The listing builds one solid part. Answer for the finished solid, in the listing's coordinates (mm). A direction names the side the tool comes from. Round coordinates to 2 decimals unless told otherwise and drop trailing zeros. Order: outer loops, then holes, each group sorted by start corner. A loop starts at its lowest first (then second) coordinate and runs counter-clockwise, first axis right, second up. Notation, with made-up numbers: (-23, 9) - (-16, 9) arc R19 cw to (-16, 13) - close; hole circle Ø9 at (-4.5, 13). An arc over 180 degrees is marked (long way). Write item = value, one per line.
from build123d import *

# Parameters (mm, degrees)
F0_R      = 2.25
F1_DEPTH  = 10
F3_DEPTH  = 20
F4_R      = 2.25
F5_DEPTH  = 5
F6_R      = 2.01
F7_DEPTH  = 5
F8_R      = 3.75
F9_DEPTH  = 2
F10_R     = 3.75
F11_DEPTH = 2


with BuildPart() as f1:
    # F0 (on Top) → F1 (new body)
    with BuildSketch(Plane.XY):
        Polygon((28.65822, 18.559446), (28.65822, -1.440554), (48.65822, -1.440554), (68.65822, -21.440554), (88.65822, -21.440554), (88.65822, -1.440554), (68.65822, -1.440554), (68.65822, 18.559446), align=None)
        with Locations((43.65822, 8.559446)):
            Circle(F0_R, mode=Mode.SUBTRACT)
        with Locations((58.65822, 8.559446)):
            Circle(F0_R, mode=Mode.SUBTRACT)
    extrude(amount=F1_DEPTH)

    # F2 (on face) → F3 (join)
    with BuildSketch(Plane.XY.offset(10)):
        Polygon((68.65822, -21.440554), (68.65822, -1.440554), (48.65822, -1.440554), (53.65822, -6.440554), (58.65822, -6.440554), (63.65822, -6.440554), (63.65822, -11.440554), (63.65822, -16.440554), align=None)
    extrude(amount=F3_DEPTH)

    # F4 (on face) → F5 (cut)
    with BuildSketch(Plane.YZ.offset(68.65822)):
        with Locations((-14.440554, 20)):
            Circle(F4_R)
    extrude(amount=-F5_DEPTH, mode=Mode.SUBTRACT)

    # F6 (on face) → F7 (cut)
    with BuildSketch(Plane(origin=(0, -1.440554, 0), x_dir=(-1, 0, 0), z_dir=(0, 1, 0))):
        with Locations((-55.65822, 20)):
            Circle(F6_R)
    extrude(amount=-F7_DEPTH, mode=Mode.SUBTRACT)

    # F8 (on face) → F9 (cut)
    with BuildSketch(Plane(origin=(63.65822, 0, 0), x_dir=(0, -1, 0), z_dir=(-1, 0, 0))):
        with Locations((14.440554, 20)):
            Circle(F8_R)
    extrude(amount=-F9_DEPTH, mode=Mode.SUBTRACT)

    # F10 (on face) → F11 (cut)
    with BuildSketch(Plane.XZ.offset(6.440554)):
        with Locations((55.65822, 20)):
            Circle(F10_R)
    extrude(amount=-F11_DEPTH, mode=Mode.SUBTRACT)


solid = f1.part
Q1. Determine the mould class of faces 4 (the face through (62, -6, 30)), 5 (the face through (64.644, -10.694, 20.165)), 6 (the face through (59, -1.441, 20)) for opening direction Y: released by +Y, released by -Y, zero draft, split by the parting line, or undercut.
Model answer:
face_4 = zero draft
face_5 = undercut
face_6 = released by +Y
Q2. Flat-ended cylindrical pins translate along their axes: P1, Ø1.5, axis at y = -9.5, z = 13, coming from the -X side; P2, Ø6, axis at x = 56.5, z = 20, coming from the -Y side; P3, Ø6, axis at y = -7.5, z = 19.5, coming from the +X side; P4, Ø6, axis at x = 54.5, y = -15.5, coming from the -Z side. Find the tip coordinate at first contact, or state that the pin passes through.
Model answer:
P1 = 63.66
P2 = -6.44
P3 = 68.66
P4 = through
Q3. For faces 1 (the face through (79, -1.441, 5)), 2 (the face through (39, -1.441, 5)), 3 (the face through (61, -9, 10)), determine the directions among +Z, -Z, +X, -X, +Y, -Y from which every point of the face is accessible in a straight line to the end or side of a thin tool.
Model answer:
face_1 = +Z, -Z, +X, +Y
face_2 = +Z, -Z, -X, -Y
face_3 = +Z, -X, -Y
Q4. Section A-A on z = 20 is taken. Determine the outline of the cut face in (x, y).
Model answer:
outline = (48.66, -1.44) - (51.91, -4.69) - (51.91, -4.44) - (53.65, -4.44) - (53.65, -1.44) - close; (57.67, -4.44) - (59.41, -4.44) - (59.41, -6.44) - (63.66, -6.44) - (63.66, -10.69) - (65.66, -10.69) - (65.66, -12.19) - (68.66, -12.19) - (68.66, -1.44) - (57.67, -1.44) - close; (65.41, -18.19) - (68.66, -21.44) - (68.66, -16.69) - (65.66, -16.69) - (65.66, -18.19) - close
Q5. Section C-C on z = 26.5 is taken. Determine the outline of the cut face in (x, y).
Model answer:
outline = (48.66, -1.44) - (53.66, -6.44) - (63.66, -6.44) - (63.66, -16.44) - (68.66, -21.44) - (68.66, -1.44) - close
Q6. Section B-B on x = 42.5 is taken. Determine the outline of the cut face in (y, z), then the cut area to 3 significant figures.
Model answer:
outline = (-1.44, 0) - (6.63, 0) - (6.63, 10) - (-1.44, 10) - close; (10.49, 0) - (18.56, 0) - (18.56, 10) - (10.49, 10) - close
area = 161 mm^2
Q7. Find the intervals of material crossed by line 1 (Y direction, x = 55, z = 23.5); line 2 (X direction, y = -5.45, z = 20); line 3 (Y direction, x = 37.5, z = 7), in increasing order. Write a range as from..to.
Model answer:
line_1 = -4.44..-1.44
line_2 = 59.41..68.66
line_3 = -1.44..18.56
Q8. Section D-D on y = -3.5 is taken. Determine the outline of the cut face in (x, z).
Model answer:
outline = (50.72, 0) - (88.66, 0) - (88.66, 10) - (68.66, 10) - (68.66, 30) - (50.72, 30) - close; hole circle Ø4.02 at (55.66, 20)
